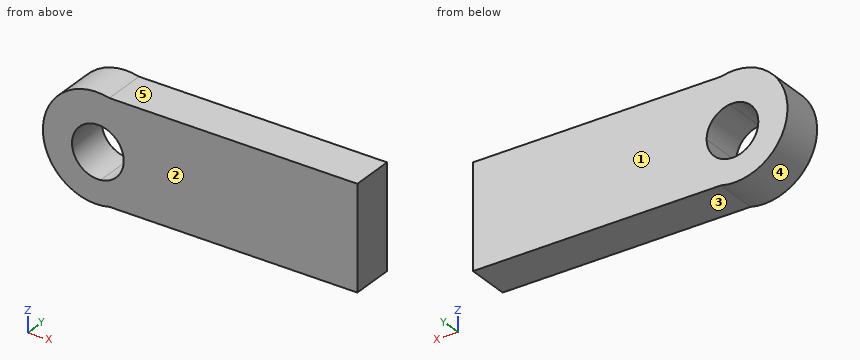
from build123d import *

# Parameters (mm, degrees)
F1_DEPTH = 25.4
F3_DEPTH = 25.4


# Not quite as in the source:
# - a feature names something its author has since deleted; it is built from what else it names


with BuildPart() as f1:
    # F0 (on Front) → F1 (new body)
    with BuildSketch(Plane.XZ):
        with BuildLine():
            Line((75.9890973568, -30.600361526), (75.9890973568, 30.600361526))
            Line((75.9890973568, 30.600361526), (-70.8035532623, 30.600361526))
            ThreePointArc((-70.8035532623, 30.600361526), (-53.6695268316, 19.3760533103), (-47.026597149, 0))
            ThreePointArc((-47.026597149, 0), (-53.6695268316, -19.3760533103), (-70.8035532623, -30.600361526))
            Line((-70.8035532623, -30.600361526), (75.9890973568, -30.600361526))
        make_face()
    extrude(amount=F1_DEPTH)

    # F0 (on Front) → F3 (join)
    with BuildSketch(Plane.XZ):
        with BuildLine():
            Line((75.9890973568, -30.600361526), (75.9890973568, 30.600361526))
            Line((75.9890973568, 30.600361526), (-70.8035532623, 30.600361526))
            ThreePointArc((-70.8035532623, 30.600361526), (-53.6695268316, 19.3760533103), (-47.026597149, 0))
            ThreePointArc((-47.026597149, 0), (-53.6695268316, -19.3760533103), (-70.8035532623, -30.600361526))
            Line((-70.8035532623, -30.600361526), (75.9890973568, -30.600361526))
        make_face()
        with BuildLine():
            ThreePointArc((-47.026597149, 0), (-53.6695268316, 19.3760533103), (-70.8035532623, 30.600361526))
            Line((-70.8035532623, 30.600361526), (-75.9890973568, 30.600361526))
            Line((-75.9890973568, 30.600361526), (-75.9890973568, 13.2593563534))
            ThreePointArc((-75.9890973568, 13.2593563534), (-66.2306105471, 8.26762835), (-62.3079244328, -1.9675046206))
            ThreePointArc((-62.3079244328, -1.9675046206), (-66.2306105471, -12.2026375911), (-75.9890973568, -17.1943655945))
            Line((-75.9890973568, -17.1943655945), (-75.9890973568, -30.600361526))
            Line((-75.9890973568, -30.600361526), (-70.8035532623, -30.600361526))
            ThreePointArc((-70.8035532623, -30.600361526), (-53.6695268316, -19.3760533103), (-47.026597149, 0))
        make_face()
        with BuildLine():
            Line((-75.9890973568, 30.600361526), (-70.8035532623, 30.600361526))
            ThreePointArc((-70.8035532623, 30.600361526), (-110.1854708241, 0), (-70.8035532623, -30.600361526))
            Line((-70.8035532623, -30.600361526), (-75.9890973568, -30.600361526))
            Line((-75.9890973568, -30.600361526), (-75.9890973568, -17.1943655945))
            ThreePointArc((-75.9890973568, -17.1943655945), (-92.9362769889, -1.9675046206), (-75.9890973568, 13.2593563534))
            Line((-75.9890973568, 13.2593563534), (-75.9890973568, 30.600361526))
        make_face()
    extrude(amount=F3_DEPTH)


solid = f1.part
Work out the finished part from the listing and answer in its coordinate system (mm). Face numbers are marked on the shaded views. A direction names the side the tool comes from. Round coordinates to 2 decimals unless told otherwise and drop trailing zeros. Loops run counter-clockwise (first coordinate to the right, second up) from the corner with the lowest first, then second, coordinate; pieces in that order, holes last. Notation, with made-up numbers: M -7.75,83.5 L 33.25,83.5 A23 cw 33.25,115.5 Z; hole C 87,64 d4. An arc over 180 degrees is marked long. One line per question, with ' | ' between items. Start each with the question number.
(1) Find the intervals of material crossed by line 1 (Z direction, x = 20, y = -1.75); line 2 (Z direction, x = -68, y = -4.5); line 3 (X direction, y = -5, z = -11.5), in increasing order.
(2) A cutting plane is placed at A-A on z = 0. Write down the section's boundary in (x, y), plus the area to 3 significant figures.
(3) For a pull along Y with two mould halves and no side action, classify the marked faces 1, 2 and 3 as released by +Y, released by -Y, zero draft, split by the parting line, or undercut.
(4) A cutting plane is placed at B-B on y = -4.5. Write down the section's boundary in (x, z), plus the area to 3 significant figures.
(5) A cutting plane is placed at D-D on x = -45.5. Write down the section's boundary in (y, z).
(6) Flat-ended cylindrical pins translate along their axes: pin 1 Ø12.5 at (x, y) = (-28, -18.5) entering from +Z; pin 2 Ø8 at (x, z) = (-69.5, -8) entering from -Y; pin 3 Ø5 at (x, z) = (53, 0) entering from +Y; pin 4 Ø5 at (y, z) = (-10.5, 24) entering from -X. Find the tip coordinate at first contact, or state that the pin passes through.
(7) A cutting plane is placed at C-C on x = -80. Write down the section's boundary in (y, z).
(8) A tool of negligible diameter and unlimited length cuts with its end or side. For the marked faces 4 and 5, from which of +Z, -Z, +X, -X, +Y, -Y can it reach the whole face along a straight path? Write none if from no direction.
Geometry check:
1) line 1: z = -30.6 to 30.6 | line 2: z = -30.6 to -13.88, 9.95 to 30.6 | line 3: x = -108.02 to -89.61, -65.64 to 75.99
2) outline: M -110.19,-25.4 L -92.81,-25.4 L -92.81,0 L -110.19,0 Z; M -62.43,-25.4 L 75.99,-25.4 L 75.99,0 L -62.43,0 Z | area: 3,960 mm²
3) face 1: released by +Y | face 2: released by -Y | face 3: zero draft
4) outline: M -70.8,-30.6 L 75.99,-30.6 L 75.99,30.6 L -70.8,30.6 A31.58 ccw long Z; hole C -77.62,-1.97 d30.63 | area: 10,300 mm²
5) outline: M -25.4,-30.6 L 0,-30.6 L 0,30.6 L -25.4,30.6 Z
6) pin 1: stops at z = 30.6 | pin 2: passes through | pin 3: stops at y = 0 | pin 4: stops at x = -101.74
7) outline: M -25.4,-31.55 L 0,-31.55 L 0,-17.1 L -25.4,-17.1 Z; M -25.4,13.16 L 0,13.16 L 0,31.55 L -25.4,31.55 Z
8) face 4: +Y, -Y | face 5: +Z, +X, +Y, -Y
